```python
from build123d import *

# Parameters (mm, degrees)
F0_R     = 19.05
F1_DEPTH = 19.05
F2_W     = 19.05
F2_H     = 50.8
F3_DEPTH = 19.05
F5_DEPTH = 19.05


with BuildPart() as f1:
    # F0 (on Right) → F1 (new body)
    with BuildSketch(Plane.YZ):
        with BuildLine():
            ThreePointArc((0, 41.148), (-29.09603, 29.09603), (-41.148, 0))
            Line((-41.148, 0), (-41.148, -111.252))
            Line((-41.148, -111.252), (-22.098, -111.252))
            Line((-22.098, -111.252), (-22.098, -60.452))
            Line((-22.098, -60.452), (22.098, -60.452))
            Line((22.098, -60.452), (22.098, -111.252))
            Line((22.098, -111.252), (41.148, -111.252))
            Line((41.148, -111.252), (41.148, 0))
            ThreePointArc((41.148, 0), (29.09603, 29.09603), (0, 41.148))
        make_face()
        Circle(F0_R, mode=Mode.SUBTRACT)
    extrude(amount=F1_DEPTH)

    # F2 (on face) → F3 (join)
    with BuildSketch(Plane.YZ.offset(19.05)):
        with Locations((-31.623, -85.852)):
            Rectangle(F2_W, F2_H)
    extrude(amount=F3_DEPTH)

    # F4 (on face) → F5 (join)
    with BuildSketch(Plane(origin=(0, 41.148, 0), x_dir=(-1, 0, 0), z_dir=(0, 1, 0))):
        Polygon((-19.05, -60.452), (-38.1, -111.252), (-19.05, -111.252), align=None)
    extrude(amount=-F5_DEPTH)


solid = f1.part
```
Geometry: final body of the model. Coordinates: model frame, mm. A direction names the side the tool comes from. Round coordinates to 2 decimals unless told otherwise and drop trailing zeros. Write each loop counter-clockwise with the first axis right and the second up, starting at its lowest first coordinate (ties: lowest second). Pieces come first, ordered by that corner, then holes.
Item 1: Section query C-C (z = -7). Return loops of the section in (x, y), plus the area to 3 significant figures.
Item 2: Set-up query: faces 4 (the face through (28.442, 31.756, -85.496)), 5 (the face through (9, 0, -60.452)), 6 (the face through (19, 32, -111.252)), 7 (the face through (28, -32, -60.452)), 8 (the face through (11, 41.148, -67)). Return all of +Z, -Z, +X, -X, +Y, -Y with unobstructed straight access to the full face (end or side cutting, diameter ignored); none if empty.
Item 3: Section query A-A (y = -12.5). Return loops of the section in (x, z), plus the area to 3 significant figures.
Item 4: Section query D-D (z = -29). Return loops of the section in (x, y).
Item 5: Section query B-B (x = 4). Return loops of the section in (y, z), plus the area to 3 significant figures.
Item 6: Pin query (flat end, axial travel): P1, Ø15, axis at x = 25, y = -33.5, coming from the +Z side; P2, Ø15, axis at x = 5.5, y = -0.5, coming from the -Z side. Return the tip coordinate at first contact, or that it passes through.
Item 7: Mould query, pull axis Y, two halves, no side actions, for faces 1 (the face through (19, -22.098, -86)), 2 (the face through (15, -41.148, -69)), 3 (the face through (19, -32, -111.252)). Classes: +Y half, -Y half, draft (parallel to the pull), parting line (faces both ways), or undercut.
Item 8: Material intervals for L1, parallel to X at y = 6, z = -34; L2, parallel to Z at x = 16, y = -8.5; L3, parallel to Z at x = 4, y = -9, sorted ascending.
Completed:
1. outline: (0, -41.15) - (19.05, -41.15) - (19.05, -17.72) - (0, -17.72) - close; (0, 17.72) - (19.05, 17.72) - (19.05, 41.15) - (0, 41.15) - close
1. area: 893 mm2
2. face 4: +Z, +X, +Y
2. face 5: -Z, +X, -X
2. face 6: -Z, +X, -X, +Y, -Y
2. face 7: +Z, +X, +Y, -Y
2. face 8: +Z, -Z, +X, -X, +Y
3. outline: (0, -60.45) - (19.05, -60.45) - (19.05, -14.38) - (0, -14.38) - close; (0, 14.38) - (19.05, 14.38) - (19.05, 39.2) - (0, 39.2) - close
3. area: 1,350 mm2
4. outline: (0, -41.15) - (19.05, -41.15) - (19.05, 41.15) - (0, 41.15) - close
5. outline: (-41.15, -111.25) - (-22.1, -111.25) - (-22.1, -60.45) - (22.1, -60.45) - (22.1, -111.25) - (41.15, -111.25) - (41.15, 0) arc R41.15 ccw to (0, 41.15) arc R41.15 ccw to (-41.15, 0) - close; hole circle Ø38.1 at (0, 0)
5. area: 8,430 mm2
6. P1: stops at z = 29.26
6. P2: stops at z = -60.45
7. face 1: undercut
7. face 2: -Y half
7. face 3: draft
8. L1: x = 0 to 19.05
8. L2: z = -60.45 to -17.05, 17.05 to 40.26
8. L3: z = -60.45 to -16.79, 16.79 to 40.15
